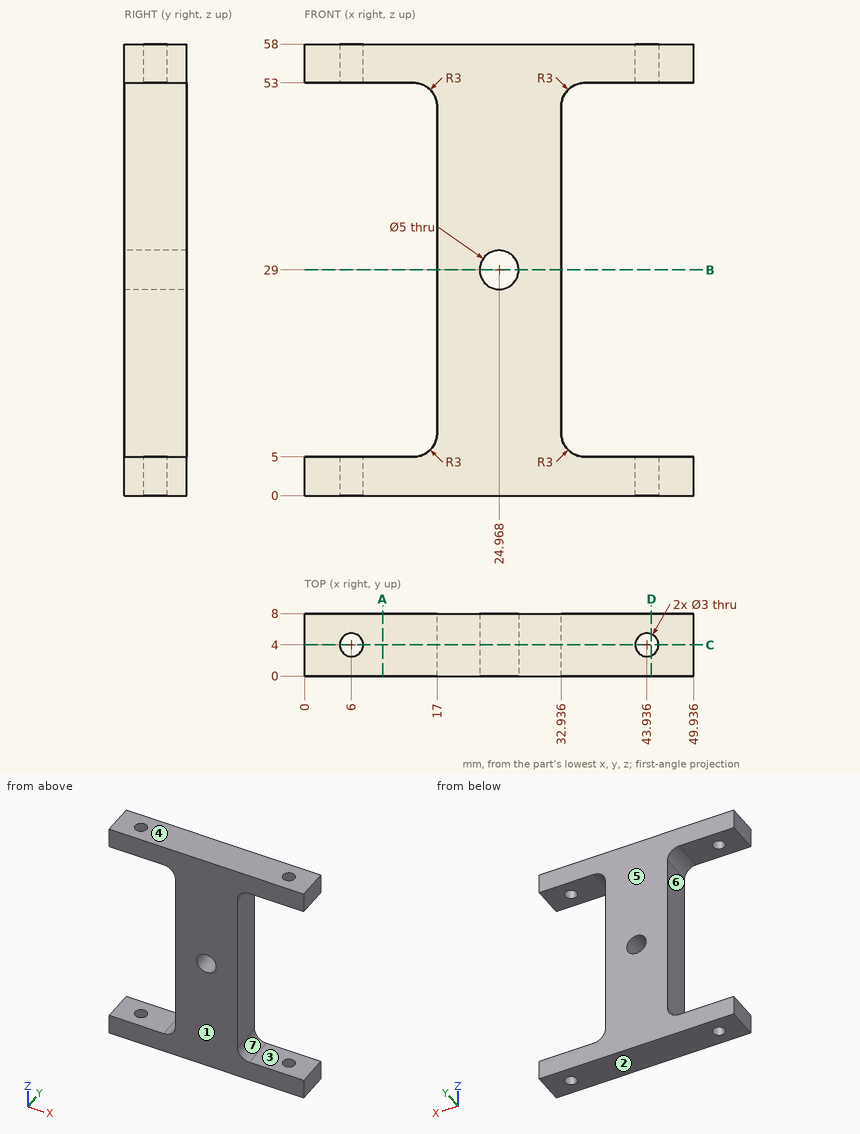
Design review of the part shown in the three views and the two pictorial views. Dimensions are in mm from the part's minimum x, y and z. A direction names the side the tool comes from. Give positions to 0.01 mm unless a question says otherwise; leave off trailing zeros. Loops run counter-clockwise (first coordinate to the right, second up) from the corner with the lowest first, then second, coordinate; pieces in that order, holes last. Notation, with made-up numbers: (59, 60.25) -> (65, 60.25) arc R14 cw to (65, 73.25) -> close; hole circle Ø5 at (-10.5, -10.75). An arc over 180 degrees is marked (long way). Answer as a JSON object with one key per item and string values. Group by question number.
Q1. Insertion check: pin 1 (3 mm diameter, centred on x = 19.5, y = 3, fed in from -Z); pin 2 (2.5 mm diameter, centred on y = 4, z = 24, fed in from -X). Each pin has a flat end and moves straight along its axis. Give the tip position at first contact, or say it passes through.
Q2. Wall thickness on line 1 along Z through (x, y) = (10, 5.75); line 2 along Y through (x, z) = (6, 57.05); line 3 along X through (y, z) = (5.5, 42.5) (1 decimal): over which ranges is each line inside the solid? List them lowest first.
Q3. Take a section at C-C (y = 4). State how many separate pieces and enclosed holes the cut face has, plus the area to 3 significant figures.
Q4. Take a section at B-B (z = 29). Write out the cut boundary in (x, y) (1 decimal).
Q5. Take a section at A-A (x = 10). Write out the cut boundary in (y, z).
Q6. Take a section at D-D (x = 44.5). Write out the cut boundary in (y, z).
Q7. Draft analysis for pull direction Z (two halves, no side actions). For the marked faces 1, 2, 3 and 4, state which applies: pulls with the +Z half, pulls with the -Z half, needs draft (parallel to the pull), parting line crosses it, or undercut.
Q8. Tool access review of the marked faces 5, 6 and 7: name each direction out of +Z, -Z, +X, -X, +Y, -Y from which nothing blocks a thin tool from reaching the whole face with its end or side.
Answer below:
{
 "1": {"pin 1": "stops at z = 0", "pin 2": "stops at x = 17"},
 "2": {"line 1": "z = 0 to 5, 53 to 58", "line 2": "y = 0 to 2.5, 5.5 to 8", "line 3": "x = 17 to 32.9"},
 "3": {"separate pieces": "5", "enclosed holes": "1", "area": "1,190 mm2"},
 "4": {"outline": "(17, 0) -> (22.5, 0) -> (22.5, 8) -> (17, 8) -> close; (27.5, 0) -> (32.9, 0) -> (32.9, 8) -> (27.5, 8) -> close"},
 "5": {"outline": "(0, 0) -> (8, 0) -> (8, 5) -> (0, 5) -> close; (0, 53) -> (8, 53) -> (8, 58) -> (0, 58) -> close"},
 "6": {"outline": "(0, 0) -> (2.61, 0) -> (2.61, 5) -> (0, 5) -> close; (0, 53) -> (2.61, 53) -> (2.61, 58) -> (0, 58) -> close; (5.39, 0) -> (8, 0) -> (8, 5) -> (5.39, 5) -> close; (5.39, 53) -> (8, 53) -> (8, 58) -> (5.39, 58) -> close"},
 "7": {"face 1": "needs draft", "face 2": "pulls with the -Z half", "face 3": "undercut", "face 4": "pulls with the +Z half"},
 "8": {"face 5": "+Z, -Z, +X, -X, +Y", "face 6": "-X, +Y, -Y", "face 7": "+X, +Y, -Y"}
}
